Can you work these out from the model? Positions are in its coordinate system, mm. A direction names the side the tool comes from. Give positions to 0.01 mm unless a question says otherwise; leave off trailing zeros. Order: outer loops, then holes, each group sorted by start corner. A loop starts at its lowest first (then second) coordinate and runs counter-clockwise, first axis right, second up. Notation, with made-up numbers: (50.5, -11.5) - (93.5, -11.5) arc R34 ccw to (93.5, 25.5) - close; hole circle Ø7 at (40, -5.75). An arc over 180 degrees is marked (long way). Answer as a JSON object with one key per item and string values.
Autodesk Inventor part; units mm, degrees
ref_plane "YZ Plane" through (0, 0, 0) normal (1, 0, 0) x (0, 1, 0)
ref_plane "XZ Plane" through (0, 0, 0) normal (0, 1, 0) x (-1, 0, 0)
ref_plane "XY Plane" through (0, 0, 0) normal (0, 0, 1) x (1, 0, 0)
sketch "TopProfile" plane through (0, 0, 0) normal (0, 0, 1) x (1, 0, 0)
  line L0 (-12.5751, 79.2329) -> (-31.9912, 61.979)
  line L1 (1.4359, 79.2329) -> (-31.9912, 61.979) construction
  line L2 (-12.5751, 79.2329) -> (1.4359, 79.2329)
  line L3 (-31.9912, 61.979) -> (0, 0)
  line L4 (1.4359, 79.2329) -> (33.4272, 17.2538)
  line L5 (0, 0) -> (33.4272, 17.2538) construction
  line L6 (14.011, 0) -> (33.4272, 17.2538)
  line L7 (0, 0) -> (14.011, 0)
  line L8 (-48.1736, 0) -> (49.6096, 0) construction
  line L9 (-10.7561, 72.9398) -> (-8.499, 74.1048)
  line L10 (-8.499, 74.1048) -> (-11.4466, 79.8154)
  line L11 (-11.4466, 79.8154) -> (-13.7036, 78.6504)
  line L12 (-13.7036, 78.6504) -> (-10.7561, 72.9398)
  line L13 (9.9349, 5.128) -> (12.192, 6.293)
  line L14 (12.192, 6.293) -> (15.1396, 0.5825)
  line L15 (15.1396, 0.5825) -> (12.8825, -0.5825)
  line L16 (12.8825, -0.5825) -> (9.9349, 5.128)
  line L17 (35.6405, 16.8421) -> (14.6869, -1.778)
  line L18 (14.6869, -1.778) -> (-1.0831, -1.778)
  line L19 (-1.0831, -1.778) -> (-34.2046, 62.3907)
  line L20 (-34.2046, 62.3907) -> (-13.2509, 81.0109)
  line L21 (-13.2509, 81.0109) -> (2.5191, 81.0109)
  line L22 (2.5191, 81.0109) -> (35.6405, 16.8421)
  point P0 (-11.1459, 79.2329)
  point P1 (-13.5549, 78.3622)
  point P2 (14.9908, 0.8707)
  point P3 (12.5818, 0)
  dimension "d0" = 37.6174
  dimension "d1" = 165.676
  dimension "d2" = 19.4161
  dimension "d3" = 69.7484
  dimension "d4" = 62.699
  dimension "d5" = 37.6174
  dimension "d6" = 165.676
  dimension "d15" = 2.54
  dimension "d16" = 1.778
extrude "CapFeature" add sketch "TopProfile" along normal blind 1.778 contours L2 L10 L9 L12 L0 | L11 L10 L2 | L0 L12 L11 | L12 L9 L10 L2 L4 L6 L14 L13 L16 L7 L3 L0 | L16 L13 L14 L6 L7 | L7 L15 L16 | L14 L15 L6 | L17 L18 L19 L20 L21 L22
extrude "WallsFeature" add sketch "TopProfile" against normal blind 7.62 contours L2 L10 L9 L12 L0 | L11 L10 L2 | L0 L12 L11 | L16 L13 L14 L6 L7 | L7 L15 L16 | L14 L15 L6 | L17 L18 L19 L20 L21 L22
fillet "SideFilletsFeature" radius 3.175 10 edges at (-31.9912, 61.979, -3.81) (0, 0, -3.81) (33.4272, 17.2538, -3.81) (1.4359, 79.2329, -3.81) (2.5191, 81.0109, -2.921) (-13.2509, 81.0109, -2.921) (-34.2046, 62.3907, -2.921) (35.6405, 16.8421, -2.921) (14.6869, -1.778, -2.921) (-1.0831, -1.778, -2.921)
properties part number "switchback-pickup-cover-6"
Q1. I'm going to push flat-ended pins straight in: pin 1 Ø4 at (y, z) = (27, -4) entering from -X; pin 2 Ø3 at (y, z) = (22, 0.5) entering from +X; pin 3 Ø5 at (y, z) = (23.5, 0) entering from +X. Where does each tip first touch, or does it pass through?
Recorded:
{"pin 1": "stops at x = -16.97", "pin 2": "stops at x = 33.75", "pin 3": "stops at x = 33.49"}
Q2. Which directions (+Z, -Z, +X, -X, +Y, -Y) give clear straight access to the entire face, cutting with the end or side of a thin tool? Please do faces 4 (the face through (11.277, 2.528, -3.757)), 5 (the face through (-33.37, 62.26, -2.86)).
Recorded:
{"face 4": "-Z", "face 5": "+Z, -Z, -X"}
Q3. If we section it at C-C, the plane x = 7: Please give me the cut outline in (y, z), then the cut area to 3 significant figures.
Recorded:
{"outline": "(-1.78, -7.62) - (0, -7.62) - (0, 0) - (68.45, 0) - (68.45, -7.62) - (72.33, -7.62) - (72.33, 1.78) - (-1.78, 1.78) - close", "area": "175 mm^2"}
Q4. If we section it at A-A, the plane z = -6.75: Please give me the cut outline in (x, y) (3 decimals), then the cut area to 3 significant figures.
Recorded:
{"outline": "(-33.073, 60.199) - (-1.97, -0.059) arc R3.175 ccw to (0.851, -1.778) - (13.48, -1.778) arc R3.175 ccw to (15.589, -0.976) - (33.797, 15.204) arc R3.175 ccw to (34.509, 19.034) - (3.406, 79.292) arc R3.175 ccw to (0.585, 81.011) - (-12.044, 81.011) arc R3.175 ccw to (-14.153, 80.209) - (-32.361, 64.029) arc R3.175 ccw to start; hole (-30.86, 59.788) - (-0.887, 1.719) arc R3.175 ccw to (1.934, 0) - (12.582, 0) - (9.935, 5.128) - (12.192, 6.293) - (14.991, 0.871) - (31.584, 15.616) arc R3.175 ccw to (32.296, 19.445) - (2.323, 77.514) arc R3.175 ccw to (-0.498, 79.233) - (-11.146, 79.233) - (-8.499, 74.105) - (-10.756, 72.94) - (-13.555, 78.362) - (-30.148, 63.617) arc R3.175 ccw to start", "area": "432 mm^2"}
Q5. We'd pull the mould along X, two halves only. Please class faces 1 (the face through (-16, 31, -4)), 2 (the face through (0, 40, 1.778)), 3 (the face through (2.257, 80.535, -2.855)): released by +X, released by -X, zero draft, split by the parting line, or undercut.
Recorded:
{"face 1": "undercut", "face 2": "zero draft", "face 3": "released by +X"}
Q6. If we section it at B-B, the plane y = 20.5: Please give me the cut outline in (x, z), then the cut area to 3 significant figures.
Recorded:
{"outline": "(-12.58, -7.62) - (-10.58, -7.62) - (-10.58, 0) - (31.75, 0) - (31.75, -7.62) - (33.75, -7.62) - (33.75, 1.78) - (-12.58, 1.78) - close", "area": "113 mm^2"}
Q7. If we section it at D-D, the plane y = 75.5: Please give me the cut outline in (x, z).
Recorded:
{"outline": "(-19.45, -7.62) - (-16.78, -7.62) - (-16.78, 0) - (-12.08, 0) - (-12.08, -7.62) - (-9.22, -7.62) - (-9.22, 0) - (3.36, 0) - (3.36, -7.62) - (5.36, -7.62) - (5.36, 1.78) - (-19.45, 1.78) - close"}
Q8. I need wall thicknesses on L1, parallel to Y at x = 12.5, z = -1.25; L2, parallel to Z at x = -22, y = 46; L3, parallel to Y at x = -20, z = -0.5. Which ranges of each line are inside material? Lowest first, please.
Recorded:
{"L1": "y = -1.78 to 0, 0.16 to 5.7, 57.8 to 61.67", "L2": "z = 0 to 1.78", "L3": "y = 34.87 to 38.75, 72.63 to 75.01"}
